from build123d import *

# Parameters (mm, degrees)
SKETCH1_W              = 210
SKETCH1_H              = 210
MAINEXTRUDE_DEPTH      = 2
SKETCH1_6_R            = 1.5
SCREWHOLES_DEPTH       = 2
ROUNDEDCORNERS_R       = 10
SKETCH2_R              = 1.05
SKETCH2_W              = 6
SKETCH2_H              = 37
SKETCH2_W_2            = 70
SKETCH2_H_2            = 35
KNOTCHES_SLIDERS_DEPTH = 4
SKETCH6_R              = 2
SKETCH6_R_2            = 0.98
PCBHOLES_DEPTH         = 4
PCBROUNDS_R            = 2


with BuildPart() as part:
    # Sketch1 → MainExtrude (new body, symmetric)
    with BuildSketch(Plane(origin=(0, 0, 0), x_dir=(1, 0, 0), z_dir=(0, 1, 0))):
        Rectangle(SKETCH1_W, SKETCH1_H)
    extrude(amount=MAINEXTRUDE_DEPTH, both=True)

    # Sketch1<6> → ScrewHoles (cut, symmetric)
    with BuildSketch(Plane(origin=(0, 0, 0), x_dir=(1, 0, 0), z_dir=(0, 1, 0))):
        with Locations((-99.833273811, 99.833273811)):
            Circle(SKETCH1_6_R)
        with Locations((-99.833273811, -99.833273811)):
            Circle(SKETCH1_6_R)
        with Locations((99.833273811, -99.833273811)):
            Circle(SKETCH1_6_R)
        with Locations((99.833273811, 99.833273811)):
            Circle(SKETCH1_6_R)
    extrude(amount=SCREWHOLES_DEPTH, both=True, mode=Mode.SUBTRACT)

    # RoundedCorners
    roundedcorners_edges = [part.edges().sort_by_distance(p)[0] for p in [
        (-105, 0, -105),
        (-105, 0, 105),
        (105, 0, 105),
        (105, 0, -105),
    ]]
    fillet(roundedcorners_edges, radius=ROUNDEDCORNERS_R)

    # Sketch2 → Knotches/Sliders (cut)
    with BuildSketch(Plane(origin=(0, 2, 0), x_dir=(1, 0, 0), z_dir=(0, 1, 0))):
        with Locations((-64.8, -96.8)):
            Circle(SKETCH2_R)
        with Locations((-64.8, -56.1)):
            Circle(SKETCH2_R)
        with Locations((-21.6, -56.1)):
            Circle(SKETCH2_R)
        with Locations((-21.6, -96.8)):
            Circle(SKETCH2_R)
        with Locations((21.6, -56.1)):
            Circle(SKETCH2_R)
        with Locations((21.6, -96.8)):
            Circle(SKETCH2_R)
        with Locations((64.8, -56.1)):
            Circle(SKETCH2_R)
        with Locations((64.8, -96.8)):
            Circle(SKETCH2_R)
        with Locations((-64.8, -76.5)):
            Rectangle(SKETCH2_W, SKETCH2_H)
        with Locations((-21.6, -76.5)):
            Rectangle(SKETCH2_W, SKETCH2_H)
        with Locations((21.6, -76.5)):
            Rectangle(SKETCH2_W, SKETCH2_H)
        with Locations((64.8, -76.5)):
            Rectangle(SKETCH2_W, SKETCH2_H)
        with BuildLine():
            Line((-54, 57.5), (-54, 66.15571123))
            ThreePointArc((-54, 66.15571123), (-50, 80), (-46, 66.15571123))
            Line((-46, 66.15571123), (-46, 57.5))
            ThreePointArc((-46, 57.5), (-50, 53.5), (-54, 57.5))
        make_face()
        with BuildLine():
            Line((46, 57.5), (46, 66.15571123))
            ThreePointArc((46, 66.15571123), (50, 80), (54, 66.15571123))
            Line((54, 66.15571123), (54, 57.5))
            ThreePointArc((54, 57.5), (50, 53.5), (46, 57.5))
        make_face()
        Rectangle(SKETCH2_W_2, SKETCH2_H_2)
    extrude(amount=-KNOTCHES_SLIDERS_DEPTH, mode=Mode.SUBTRACT)

    # Sketch6 → PCBHoles (add)
    with BuildSketch(Plane(origin=(71.684316031, -2, 14.480918484), x_dir=(1, 0, 0), z_dir=(0, -1, 0))):
        with Locations((-22.524316031, 23.519081516)):
            Circle(SKETCH6_R)
        with Locations((-22.524316031, 23.519081516)):
            Circle(SKETCH6_R_2, mode=Mode.SUBTRACT)
        with Locations((13.315683969, 23.519081516)):
            Circle(SKETCH6_R)
        with Locations((13.315683969, 23.519081516)):
            Circle(SKETCH6_R_2, mode=Mode.SUBTRACT)
        with Locations((-22.524316031, -50.750918484)):
            Circle(SKETCH6_R)
        with Locations((-22.524316031, -50.750918484)):
            Circle(SKETCH6_R_2, mode=Mode.SUBTRACT)
        with Locations((13.315683969, -50.750918484)):
            Circle(SKETCH6_R)
        with Locations((13.315683969, -50.750918484)):
            Circle(SKETCH6_R_2, mode=Mode.SUBTRACT)
    extrude(amount=PCBHOLES_DEPTH)

    # PCBRounds
    pcbrounds_edges = [part.edges().sort_by_distance(p)[0] for p in [
        (47.16, -2, 38),
        (83, -2, 38),
        (47.16, -2, -36.27),
        (83, -2, -36.27),
    ]]
    fillet(pcbrounds_edges, radius=PCBROUNDS_R)


solid = part.part
Build history of the part. All positions in model axes, mm. Round coordinates to 2 decimals unless told otherwise and drop trailing zeros. Order: outer loops, then holes, each group sorted by start corner. A loop starts at its lowest first (then second) coordinate and runs counter-clockwise, first axis right, second up. Notation, with made-up numbers: M 2,-30.5 L 9,-30.5 A34 cw 9,5.5 Z; hole C 61.25,25 d5. An arc over 180 degrees is marked long. Use CSV: the item, a comma, the result in double quotes. Start each with the question number.
(1) Drill centre lines: probe 1 along X at (y, z) = (1.15, 56.1); probe 2 along Z at (x, y) = (21.6, 0.55); probe 3 along Z at (x, y) = (49.16, -4.05). Where is each one in solid material? Low to high.
(2) Cut at C-C on z = 12.5. List the corners of the cut face in (x, y), then the cut area to 3 significant figures.
(3) Mould opens along X. For faces 1 (the face through (101.99, -0.03, -102.15)), 2 (the face through (50, 0, -80)), 3 (the face through (-102.15, 0.03, 101.99)), 4 (the face through (-50, 0, -80)) say: +X half, -X half, draft (parallel to the pull), parting line (faces both ways), or undercut.
(4) Flat gauge pin, fed straight in: P1, Ø1.8, axis at x = 85, z = -36.27, coming from the -Y side. Where does the tip first touch, or does it go through?
(5) Cut at A-A on z = -72.5. List the corners of the cut face in (x, y).
(6) Cut at B-B on x = 28.5. List the corners of the cut face in (y, z), then the cut area to 3 significant figures.
(7) Cut at D-D on x = 71.5. List the corners of the cut face in (y, z).
Findings:
1,probe 1,"x = -105 to -65.85, -63.75 to -22.65, -20.55 to 20.55, 22.65 to 63.75, 65.85 to 105"
1,probe 2,"z = -105 to -17.5, 17.5 to 55.05, 57.15 to 58, 95 to 95.75, 97.85 to 105"
1,probe 3,"z = -38.27 to -37.25, -35.29 to -34.27, 36 to 37.02, 38.98 to 40"
2,outline,"M -105,-2 L -35,-2 L -35,2 L -105,2 Z; M 35,-2 L 105,-2 L 105,2 L 35,2 Z"
2,area,"560 mm^2"
3,face 1,"+X half"
3,face 2,"undercut"
3,face 3,"-X half"
3,face 4,"undercut"
4,P1,"stops at y = -2"
5,outline,"M -105,-2 L -57.5,-2 L -57.5,2 L -105,2 Z; M -42.5,-2 L 42.5,-2 L 42.5,2 L -42.5,2 Z; M 57.5,-2 L 105,-2 L 105,2 L 57.5,2 Z"
6,outline,"M -2,-105 L 2,-105 L 2,-17.5 L -2,-17.5 Z; M -2,17.5 L 2,17.5 L 2,105 L -2,105 Z"
6,area,"700 mm^2"
7,outline,"M -2,-105 L 2,-105 L 2,105 L -2,105 Z"
